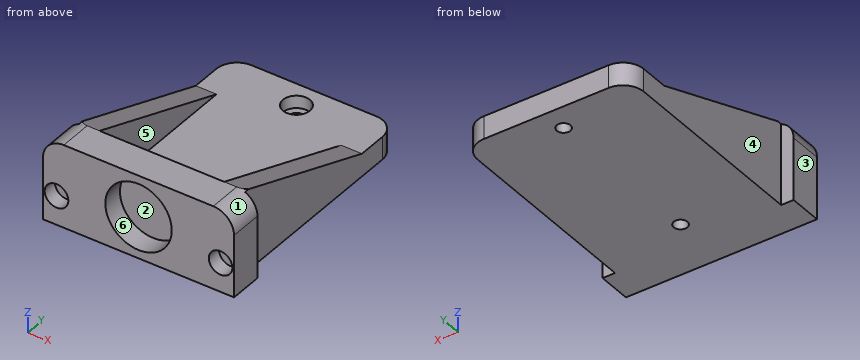
from build123d import *

# Parameters (mm, degrees)
F0_W           = 3
F0_H           = 8
F1_DEPTH       = 20
F0_W_2         = 30
F0_H_2         = 12
F0_H_3         = 40
F0_W_3         = 5
F2_DEPTH       = 5.5
F3_DEPTH       = 20
F5_DEPTH       = 43.001
F7_D           = 3.3
F7_DEPTH       = 13.5002857143
F7_CBORE_D     = 6.5
F7_CBORE_DEPTH = 3
F7_TIP         = 0.9914200214
F8_R           = 8
F9_DEPTH       = 5
F8_R_2         = 2.85
F10_DEPTH      = 3.5
F11_T1_DEPTH   = 30.5
F11_T3_DEPTH   = 33


# Not quite as in the source:
# - a fillet or chamfer that OpenCascade refuses, or shapes differently, is made with other operations: its cross-section is extruded or revolved along the edge and cut away or added


with BuildPart() as f1:
    # F0 (on Top) → F1 (new body)
    with BuildSketch(Plane.XY):
        Polygon((20, -30), (20, -22), (15, -22), (-15, -22), (-20, -22), (-20, -30), align=None)
        with Locations((-21.5, -26)):
            Rectangle(F0_W, F0_H)
        with Locations((21.5, -26)):
            Rectangle(F0_W, F0_H)
    extrude(amount=F1_DEPTH)

    # F0 (on Top) → F2 (join)
    with BuildSketch(Plane.XY):
        with Locations((0, 24)):
            Rectangle(F0_W_2, F0_H_2)
        with Locations((0, -2)):
            Rectangle(F0_W_2, F0_H_3)
        with Locations((-17.5, 24)):
            Rectangle(F0_W_3, F0_H_2)
        with Locations((-17.5, -2)):
            Rectangle(F0_W_3, F0_H_3)
        with Locations((17.5, 24)):
            Rectangle(F0_W_3, F0_H_2)
        with Locations((17.5, -2)):
            Rectangle(F0_W_3, F0_H_3)
    extrude(amount=F2_DEPTH)

    # F0 (on Top) → F3 (join)
    with BuildSketch(Plane.XY):
        with Locations((-17.5, -2)):
            Rectangle(F0_W_3, F0_H_3)
        with Locations((17.5, -2)):
            Rectangle(F0_W_3, F0_H_3)
    extrude(amount=F3_DEPTH)

    # F4 (on face) → F5 (cut, through all)
    with BuildSketch(Plane(origin=(-20, 0, 0), x_dir=(0, -1, 0), z_dir=(-1, 0, 0))):
        Polygon((-18, 20), (-18, 5.5), (22, 20), align=None)
    extrude(amount=-F5_DEPTH, mode=Mode.SUBTRACT)

    # F7
    with Locations(Plane.XY.offset(5.5)):
        with Locations((0, 24), (0, -16)):
            CounterBoreHole(F7_D / 2, F7_CBORE_D / 2, F7_CBORE_DEPTH, depth=F7_DEPTH)
            with Locations((0, 0, -(F7_DEPTH + F7_TIP / 2))):  # 118° drill point
                Cone(0, F7_D / 2, F7_TIP, mode=Mode.SUBTRACT)

    # F8 (on face) → F9 (cut)
    with BuildSketch(Plane.XZ.offset(30)):
        with Locations((0, 10)):
            Circle(F8_R)
    extrude(amount=-F9_DEPTH, mode=Mode.SUBTRACT)

    # F8 (on face) → F10 (cut)
    with BuildSketch(Plane.XZ.offset(30)):
        with Locations((-19.75, 7)):
            Circle(F8_R_2)
        with Locations((19.75, 7)):
            Circle(F8_R_2)
    extrude(amount=-F10_DEPTH, mode=Mode.SUBTRACT)

    # F11: fillet of radius 5 on 4 edges, made by hand

    # F11_s2 → F11_t1 (cut)
    with BuildSketch(Plane.XY.offset(-12.5)):
        with BuildLine():
            ThreePointArc((15, 30), (18.5355339059, 28.5355339059), (20, 25))
            Line((20, 25), (20, 30))
            Line((20, 30), (15, 30))
        make_face()
        with BuildLine():
            ThreePointArc((-20, 25), (-18.5355339059, 28.5355339059), (-15, 30))
            Line((-15, 30), (-20, 30))
            Line((-20, 30), (-20, 25))
        make_face()
    extrude(amount=F11_T1_DEPTH, mode=Mode.SUBTRACT)

    # F11_s4 → F11_t3 (cut)
    with BuildSketch(Plane.XZ.offset(9.5)):
        with BuildLine():
            ThreePointArc((-23, 15), (-21.5355339059, 18.5355339059), (-18, 20))
            Line((-18, 20), (-23, 20))
            Line((-23, 20), (-23, 15))
        make_face()
        with BuildLine():
            ThreePointArc((18, 20), (21.5355339059, 18.5355339059), (23, 15))
            Line((23, 15), (23, 20))
            Line((23, 20), (18, 20))
        make_face()
    extrude(amount=F11_T3_DEPTH, mode=Mode.SUBTRACT)


solid = f1.part
Design review of the part built by this model. Coordinates are the model's own, in mm. Face numbers are marked on the shaded views. A direction names the side the tool comes from. Give positions to 0.01 mm unless a question says otherwise; leave off trailing zeros. Order: outer loops, then holes, each group sorted by start corner. A loop starts at its lowest first (then second) coordinate and runs counter-clockwise, first axis right, second up. Notation, with made-up numbers: (-4, -11) - (14, -11) arc R16 ccw to (14, 3) - close; hole circle Ø4 at (57, 59.25). An arc over 180 degrees is marked (long way). Write item = value, one per line. Start each with the question number.
Q1. Tool access review of the marked faces 4, 5 and 6: name each direction out of +Z, -Z, +X, -X, +Y, -Y from which nothing blocks a thin tool from reaching the whole face with its end or side.
Q2. We need section C-C on x = -11. State the section outline as (y, z) points, plus the area to 3 significant figures.
Q3. To check wall thickness, follow L1, parallel to Y at x = 0, z = 4.35; L2, parallel to Y at x = 0, z = 0.5; L3, parallel to Z at x = 0, y = -28.55. State the ranges of each line that lie inside material, in increasing order. Write a range as from..to.
Q4. We need section B-B on x = 1. State the section outline as (y, z) points.
Q5. We need section A-A on y = 24. State the section outline as (x, z) points.
Q6. Mouldability with a two-part tool opening along Z and no side actions: class the marked faces 1, 2 and 3 as released by +Z, released by -Z, zero draft, split by the parting line, or undercut.
Q7. Clearance check with flat-ended pins moving along their axes: pin 1 Ø4 at (x, y) = (-12.5, 6) entering from +Z; pin 2 Ø1 at (y, z) = (-19, 13.5) entering from -X; pin 3 Ø10 at (x, z) = (-7, 11) entering from +Y. State where each tip first meets the part, or that it passes through.
Q8. We need section D-D on y = -10. State the section outline as (x, z) points, plus the area to 4 significant figures.
Working result:
q1.face_4 = +Z, -Z, -X, +Y
q1.face_5 = +Z, +Y
q1.face_6 = -Y
q2.outline = (-30, 0) - (30, 0) - (30, 5.5) - (-22, 5.5) - (-22, 20) - (-30, 20) - close
q2.area = 446 mm²
q3.L1 = -25..-19.25, -12.75..20.75, 27.25..30
q3.L2 = -30..-17.65, -14.35..22.35, 25.65..30
q3.L3 = 0..2, 18..20
q4.outline = (-30, 0) - (-17.31, 0) - (-17.31, 2.5) - (-19.09, 2.5) - (-19.09, 5.5) - (-22, 5.5) - (-22, 20) - (-30, 20) - (-30, 17.94) - (-25, 17.94) - (-25, 2.06) - (-30, 2.06) - close; (-14.69, 0) - (22.69, 0) - (22.69, 2.5) - (20.91, 2.5) - (20.91, 5.5) - (-12.91, 5.5) - (-12.91, 2.5) - (-14.69, 2.5) - close; (25.31, 0) - (30, 0) - (30, 5.5) - (27.09, 5.5) - (27.09, 2.5) - (25.31, 2.5) - close
q5.outline = (-20, 0) - (-1.65, 0) - (-1.65, 2.5) - (-3.25, 2.5) - (-3.25, 5.5) - (-20, 5.5) - close; (1.65, 0) - (20, 0) - (20, 5.5) - (3.25, 5.5) - (3.25, 2.5) - (1.65, 2.5) - close
q6.face_1 = released by +Z
q6.face_2 = undercut
q6.face_3 = zero draft
q7.pin_1 = 5.5
q7.pin_2 = -20
q7.pin_3 = -22
q8.outline = (-20, 0) - (20, 0) - (20, 15.65) - (15, 15.65) - (15, 5.5) - (-15, 5.5) - (-15, 15.65) - (-20, 15.65) - close
q8.area = 321.5 mm²
